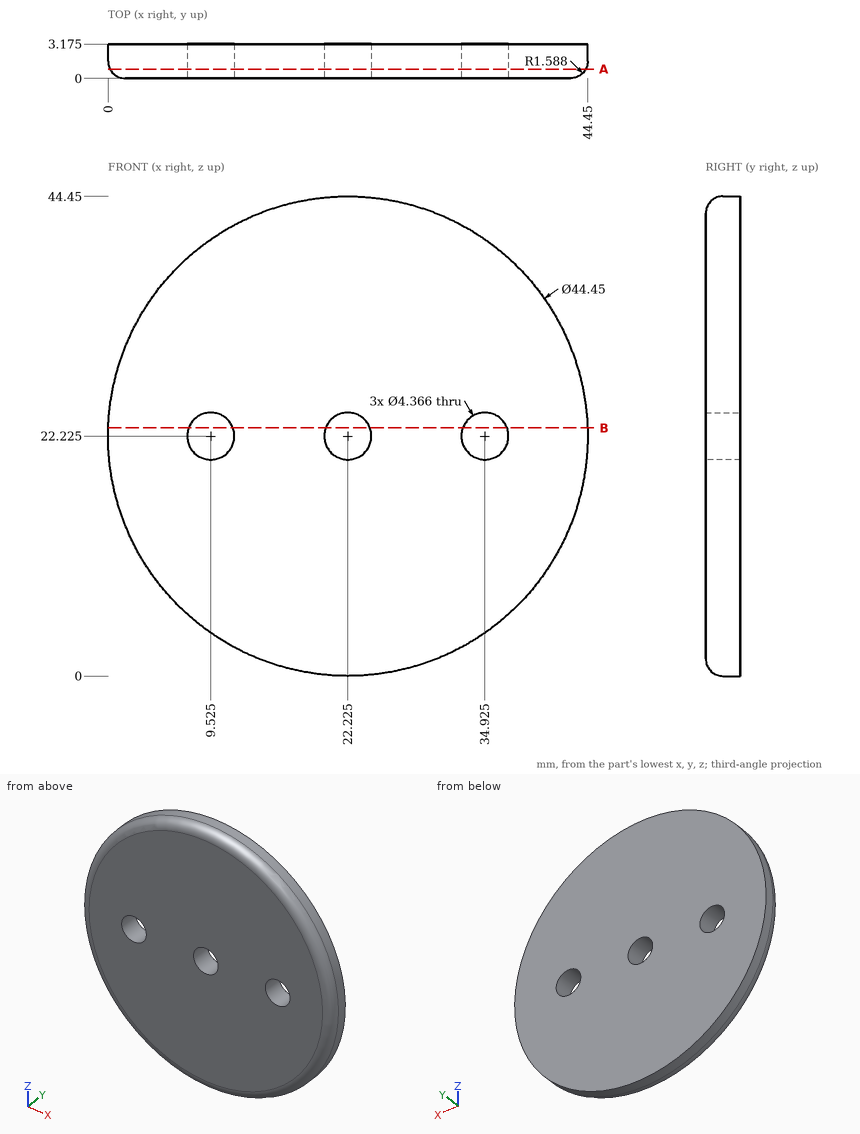
Source: three-view drawing plus pictorial views. Frame: mm from the lowest corner of the part. Give positions to 0.01 mm unless a question says otherwise; leave off trailing zeros. Write each loop counter-clockwise with the first axis right and the second up, starting at its lowest first coordinate (ties: lowest second). Pieces come first, ordered by that corner, then holes. Notation, with made-up numbers: (-26, 76.5) - (-20, 76.5) arc R8 ccw to (-20, 91.5) - close; hole circle Ø3 at (-30.5, 29). An arc over 180 degrees is marked (long way). Write item = value, one per line. Start each with the question number.
1. Section query A-A, the plane y = 0.85. Output: boundary loops of the cut face in (x, z) (1 decimal), then the cut area to 3 significant figures.
2. Ray query, L1, parallel to X at y = 0.7, z = 21 (1 decimal); L2, parallel to Z at x = 9.5, y = 2.55 (1 decimal); L3, parallel to Z at x = 30.5, y = 2.95. Return the intervals inside material, ascending.
3. Section query B-B, the plane z = 23. Count the separate pieces of the cut face and the enclosed holes in it, then the cut area to 3 significant figures.
Check sheet entries:
q1.outline = circle Ø44.1 at (22.2, 22.2); hole circle Ø4.4 at (9.5, 22.2); hole circle Ø4.4 at (22.2, 22.2); hole circle Ø4.4 at (34.9, 22.2)
q1.area = 1,480 mm2
q2.L1 = 0.3 to 7.7, 11.3 to 20.4, 24 to 33.1, 36.7 to 44.1
q2.L2 = 4 to 20, 24.4 to 40.4
q2.L3 = 1.6 to 42.85
q3.separate_pieces = 4
q3.enclosed_holes = 0
q3.area = 101 mm2
